```python
from build123d import *

# Parameters (mm, degrees)
SKETCH_1_W                  = 18
SKETCH_1_H                  = 9
EXTRUDE_1_DEPTH             = 6
SKETCH_2_W                  = 24
SKETCH_2_H                  = 9
EXTRUDE_2_DEPTH             = 1
FILLET_1_R                  = 1
CHAMFER_1_SIZE              = 0.5
CHAMFER_2_SIZE              = 0.2
HOLE_WIZARD_M2_1_AT_2_COUNT = 2
HOLE_WIZARD_M2_1_AT_2_PITCH = 6.4
HOLE_WIZARD_M2_1_AT_3_COUNT = 2
HOLE_WIZARD_M2_1_AT_3_PITCH = 22.336517186
HOLE_WIZARD_M2_1_AT_4_COUNT = 2
HOLE_WIZARD_M2_1_AT_4_PITCH = 21.4


with BuildPart() as part:
    # 草图1 → 凸台-拉伸1 (new body)
    with BuildSketch(Plane(origin=(0, 0, 0), x_dir=(1, 0, 0), z_dir=(0, 1, 0))):
        Rectangle(SKETCH_1_W, SKETCH_1_H)
    extrude(amount=EXTRUDE_1_DEPTH)

    # 草图2 → 凸台-拉伸2 (add)
    with BuildSketch(Plane(origin=(0, 6, 0), x_dir=(1, 0, 0), z_dir=(0, 1, 0))):
        Rectangle(SKETCH_2_W, SKETCH_2_H)
    extrude(amount=EXTRUDE_2_DEPTH)

    # 圆角1
    fillet_1_edges = [part.edges().sort_by_distance(p)[0] for p in [
        (-12, 6.5, -4.5),
        (-12, 6.5, 4.5),
        (12, 6.5, 4.5),
        (12, 6.5, -4.5),
    ]]
    fillet(fillet_1_edges, radius=FILLET_1_R)

    # 倒角1
    chamfer_1_edges = [part.edges().sort_by_distance(p)[0] for p in [
        (0, 0, -4.5),
        (9, 0, 0),
        (0, 0, 4.5),
        (-9, 0, 0),
    ]]
    chamfer(chamfer_1_edges, length=CHAMFER_1_SIZE)

    # 倒角2
    chamfer_2_edges = [part.edges().sort_by_distance(p)[0] for p in [
        (-9, 3.25, -4.5),
        (9, 3.25, -4.5),
        (9, 3.25, 4.5),
        (-9, 3.25, 4.5),
    ]]
    chamfer(chamfer_2_edges, length=CHAMFER_2_SIZE)

    # 草图5 → M2 螺纹孔1 (revolve, cut)
    with BuildSketch(Plane(origin=(-10.7, 6, -3.2), x_dir=(0, 0, -1), z_dir=(1, 0, 0))):
        Polygon((0, 0), (0, 1), (0.8, 1), (0.8, 0.225), (1.025, 0), align=None)
    hole_wizard_m2_1 = revolve(axis=Axis((-10.7, -0.35, -3.2), (0, 1, 0)), mode=Mode.SUBTRACT)

    # M2 螺纹孔1 at 2: M2 螺纹孔1 ×2
    with Locations(*[(0, 0, i * HOLE_WIZARD_M2_1_AT_2_PITCH) for i in range(1, HOLE_WIZARD_M2_1_AT_2_COUNT)]):
        add(hole_wizard_m2_1, mode=Mode.SUBTRACT)

    # M2 螺纹孔1 at 3: M2 螺纹孔1 ×2
    with Locations(*[Vector(0.958072371883615, 0, 0.2865263168250065) * (i * HOLE_WIZARD_M2_1_AT_3_PITCH) for i in range(1, HOLE_WIZARD_M2_1_AT_3_COUNT)]):
        add(hole_wizard_m2_1, mode=Mode.SUBTRACT)

    # M2 螺纹孔1 at 4: M2 螺纹孔1 ×2
    with Locations(*[(i * HOLE_WIZARD_M2_1_AT_4_PITCH, 0, 0) for i in range(1, HOLE_WIZARD_M2_1_AT_4_COUNT)]):
        add(hole_wizard_m2_1, mode=Mode.SUBTRACT)


solid = part.part
```
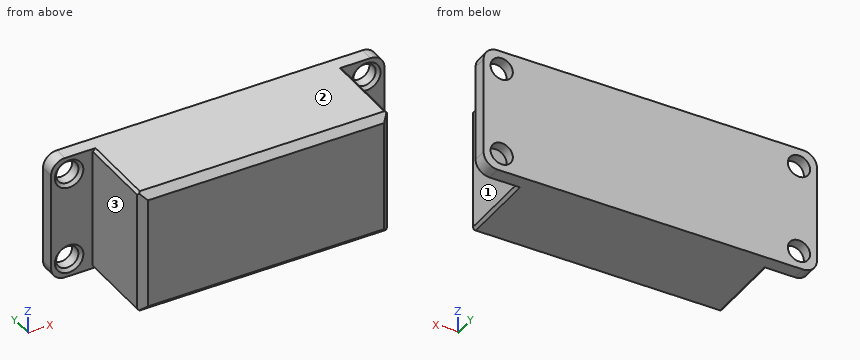
Here's how the part is built. I have some questions about the finished solid (model axes, mm). Face numbers are marked on the shaded views. A direction names the side the tool comes from. Coordinates: 2 decimals unless noted, no trailing zeros. Write each loop counter-clockwise with the first axis right and the second up, starting at its lowest first coordinate (ties: lowest second). Pieces come first, ordered by that corner, then holes. Notation, with made-up numbers: (12, 58.5) - (53, 58.5) arc R25 ccw to (53, 86.5) - close; hole circle Ø10 at (89.5, 37). An arc over 180 degrees is marked (long way). One line per item, written item: value.
1) Suppose I cut it at D-D on y = 2.5. Write out the boundary of the cut face in (x, z).
Model answer:
outline: (-9, -4.3) - (-8.8, -4.5) - (8.8, -4.5) - (9, -4.3) - (9, 4.3) - (8.8, 4.5) - (-8.8, 4.5) - (-9, 4.3) - close
2) Suppose I cut it at B-B on z = -3.2. Write out the boundary of the cut face in (x, y) (3 decimals), and give its area (3 significant figures).
Model answer:
outline: (-12, 6) - (-11.725, 6) - (-11.5, 6.225) - (-11.5, 7) - (-12, 7) - close; (-9.9, 6.225) - (-9.675, 6) - (-9, 6) - (-9, 0.5) - (-8.5, 0) - (8.5, 0) - (9, 0.5) - (9, 6) - (9.675, 6) - (9.9, 6.225) - (9.9, 7) - (-9.9, 7) - close; (11.5, 6.225) - (11.725, 6) - (12, 6) - (12, 7) - (11.5, 7) - close
area: 128 mm²
3) I'm going to push flat-ended pins straight in: P1, Ø3.5, axis at x = -11, z = 2, coming from the -Y side; P2, Ø1.3, axis at x = 10.7, z = -3.2, coming from the +Y side; P3, Ø3.5, axis at x = 10.5, z = 0, coming from the -Y side; P4, Ø4, axis at y = 2, z = -0.5, coming from the -X side. Where does each tip first touch, or does it pass through?
Model answer:
P1: stops at y = 6
P2: passes through
P3: stops at y = 0.25
P4: stops at x = -9
4) Suppose I cut it at C-C on y = 6.5. Write out the boundary of the cut face in (x, z), and give its area (3 significant figures).
Model answer:
outline: (-12, -3.5) arc R1 ccw to (-11, -4.5) - (11, -4.5) arc R1 ccw to (12, -3.5) - (12, 3.5) arc R1 ccw to (11, 4.5) - (-11, 4.5) arc R1 ccw to (-12, 3.5) - close; hole circle Ø1.6 at (-10.7, -3.2); hole circle Ø1.6 at (-10.7, 3.2); hole circle Ø1.6 at (10.7, -3.2); hole circle Ø1.6 at (10.7, 3.2)
area: 207 mm²
5) I need wall thicknesses on line 1 along X through (y, z) = (6.4, -3.2); line 2 along Z through (x, y) = (-10.7, 6.65); line 3 along X through (y, z) = (3.75, 4). Which ranges of each line are inside material? Lowest first, please.
Model answer:
line 1: x = -12 to -11.5, -9.9 to 9.9, 11.5 to 12
line 2: z = -4.5 to -4, -2.4 to 2.4, 4 to 4.5
line 3: x = -9 to 9
6) Suppose I cut it at A-A on x = -10.7. Write out the boundary of the cut face in (y, z) (3 decimals).
Model answer:
outline: (6, -4.5) - (7, -4.5) - (7, -4) - (6.225, -4) - (6, -4.225) - close; (6, -2.175) - (6.225, -2.4) - (7, -2.4) - (7, 2.4) - (6.225, 2.4) - (6, 2.175) - close; (6, 4.225) - (6.225, 4) - (7, 4) - (7, 4.5) - (6, 4.5) - close
7) On a 3-axis mill with a long thin cutter (end or side, diameter ignored), from which of +Z, -Z, +X, -X, +Y, -Y can I reach the whole of each face in a straight line? I mean the marked faces 1, 2 and 3. Say none if no direction works.
Model answer:
face 1: +Z, -Z, +X, -Y
face 2: +Z, +X, -X, +Y, -Y
face 3: +Z, -Z, -X, -Y
